```python
from build123d import *

# Parameters (mm, degrees)
F0_W     = 68
F0_H     = 25
F1_DEPTH = 3
F2_W     = 5
F2_H     = 3
F3_DEPTH = 3
F4_W     = 15
F4_H     = 3
F5_DEPTH = 3
F7_R     = 1.5
F8_DEPTH = 3


# Not quite as in the source:
# - a feature names something its author has since deleted; it is built from what else it names


with BuildPart() as f1:
    # F0 (on Top) → F1 (new body)
    with BuildSketch(Plane.XY):
        Rectangle(F0_W, F0_H)
    extrude(amount=F1_DEPTH)

    # F2 (on face) → F3 (join)
    with BuildSketch(Plane.XZ.offset(12.5)):
        with Locations((7.5, 1.5)):
            Rectangle(F2_W, F2_H)
    extrude(amount=F3_DEPTH)

    # F4 (on face) → F5 (join)
    with BuildSketch(Plane.YZ.offset(34)):
        with Locations((-5, 1.5)):
            Rectangle(F4_W, F4_H)
    extrude(amount=F5_DEPTH)

    # F6: F1 across plane


with BuildPart() as f1_1:
    add(f1.part)
    add(f1.part.mirror(Plane.YZ))

    # F7 (on face) → F8 (cut)
    with BuildSketch(Plane.XY.offset(3)):
        with Locations((22, 5)):
            Circle(F7_R)
        with Locations((-22, 5)):
            Circle(F7_R)
    extrude(amount=-F8_DEPTH, mode=Mode.SUBTRACT)


solid = f1_1.part
```
The listing builds one solid part. Answer for the finished solid, in the listing's coordinates (mm). A direction names the side the tool comes from. Coordinates: 2 decimals unless noted, no trailing zeros. Write each loop counter-clockwise with the first axis right and the second up, starting at its lowest first coordinate (ties: lowest second). Pieces come first, ordered by that corner, then holes. Notation, with made-up numbers: (73, 37) -> (126, 37) arc R18 cw to (126, 56) -> close; hole circle Ø7 at (53.5, 87). An arc over 180 degrees is marked (long way). Write each question's results on one line, items separated by ' | '. Start each with the question number.
1) A cutting plane is placed at B-B (x = 22). Determine the outline of the cut face in (y, z).
2) Flat-ended cylindrical pins translate along their axes: pin 1 Ø0.9 at (x, z) = (-1.5, 2) entering from -Y; pin 2 Ø3.5 at (x, y) = (22, 5) entering from +Z; pin 3 Ø0.9 at (y, z) = (-14, 1) entering from -X; pin 4 Ø0.9 at (y, z) = (-13.5, 1.5) entering from +X. Find the tip coordinate at first contact, or state that the pin passes through.
3) A cutting plane is placed at C-C (z = 1.25). Determine the outline of the cut face in (x, y).
4) Straight lines are drawn through the part: probe 1 along Y at (x, z) = (22, 2.25); probe 2 along X at (y, z) = (4, 1.2); probe 3 along Y at (x, z) = (28.5, 0.85). For each, find the intervals that lie inside material, in ascending order.
5) A tool of negligible diameter and unlimited length cuts with its end or side. For faces 5 (the flat face through (5, -14, 1)), 6 (the flat face through (-35, 2.5, 1)), 7 (the flat face through (23, -12.5, 1)), 8 (the flat face through (-23, -12.5, 1)), from which of +Z, -Z, +X, -X, +Y, -Y can it reach the whole face along a straight path? Write none if from no direction.
6) For a pull along X with two mould halves and no side action, classify faces 1 (the cylindrical face through (-23.5, 5.07, 1.52)), 2 (the flat face through (10, -14, 1)), 3 (the flat face through (-5, -14, 1)), 4 (the flat face through (1, -2, 0)) as +X half, -X half, draft (parallel to the pull), parting line (faces both ways), or undercut.
7) A cutting plane is placed at D-D (y = 5). Determine the outline of the cut face in (x, z).
8) A cutting plane is placed at A-A (y = -13.25). Determine the outline of the cut face in (x, z), then the cut area to 3 significant figures.
Values follow:
1) outline: (-12.5, 0) -> (3.5, 0) -> (3.5, 3) -> (-12.5, 3) -> close; (6.5, 0) -> (12.5, 0) -> (12.5, 3) -> (6.5, 3) -> close
2) pin 1: y = -12.5 | pin 2: z = 3 | pin 3: x = -10 | pin 4: x = 10
3) outline: (-37, -12.5) -> (-10, -12.5) -> (-10, -15.5) -> (-5, -15.5) -> (-5, -12.5) -> (5, -12.5) -> (5, -15.5) -> (10, -15.5) -> (10, -12.5) -> (37, -12.5) -> (37, 2.5) -> (34, 2.5) -> (34, 12.5) -> (-34, 12.5) -> (-34, 2.5) -> (-37, 2.5) -> close; hole circle Ø3 at (-22, 5); hole circle Ø3 at (22, 5)
4) probe 1: -12.5 to 3.5, 6.5 to 12.5 | probe 2: -34 to -23.12, -20.88 to 20.88, 23.12 to 34 | probe 3: -12.5 to 12.5
5) face 5: +Z, -Z, -Y | face 6: +Z, -Z, -X, +Y | face 7: +Z, -Z, +X, -Y | face 8: +Z, -Z, -X, -Y
6) face 1: undercut | face 2: +X half | face 3: undercut | face 4: draft
7) outline: (-34, 0) -> (-23.5, 0) -> (-23.5, 3) -> (-34, 3) -> close; (-20.5, 0) -> (20.5, 0) -> (20.5, 3) -> (-20.5, 3) -> close; (23.5, 0) -> (34, 0) -> (34, 3) -> (23.5, 3) -> close
8) outline: (-10, 0) -> (-5, 0) -> (-5, 3) -> (-10, 3) -> close; (5, 0) -> (10, 0) -> (10, 3) -> (5, 3) -> close | area: 30.0 mm²
